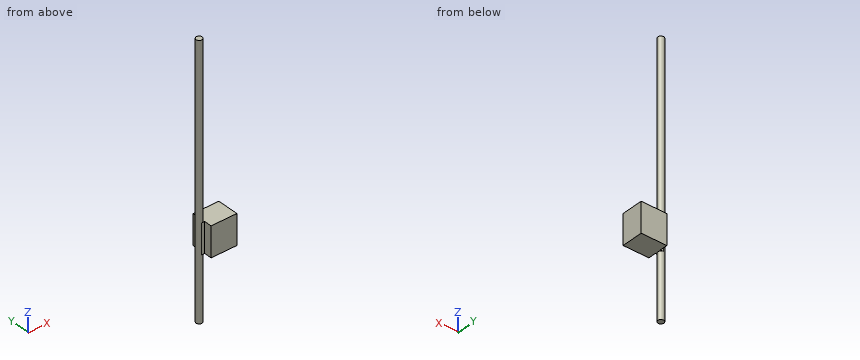
```python
from build123d import *

# Parameters (mm, degrees)
F0_R     = 17.78
F1_DEPTH = 787.4
F2_W     = 152.4
F2_H     = 177.8
F3_DEPTH = 63.5
F5_DEPTH = 177.8


with BuildPart() as f1:
    # F0 (on Top) → F1 (new body, symmetric)
    with BuildSketch(Plane.XY):
        Circle(F0_R)
    extrude(amount=F1_DEPTH, both=True)

    # F2 (on Front) → F3 (join, symmetric)
    with BuildSketch(Plane.XZ):
        with Locations((93.98, -317.5)):
            Rectangle(F2_W, F2_H)
    extrude(amount=F3_DEPTH, both=True)

    # F4 (on face) → F5 (join, through all)
    with BuildSketch(Plane.XY.offset(-228.6)):
        with BuildLine():
            Line((17.78, -17.78), (17.78, 0))
            ThreePointArc((17.78, 0), (12.5723585695, -12.5723585695), (0, -17.78))
            Line((0, -17.78), (17.78, -17.78))
        make_face()
        with BuildLine():
            ThreePointArc((0, 17.78), (12.5723585695, 12.5723585695), (17.78, 0))
            Line((17.78, 0), (17.78, 17.78))
            Line((17.78, 17.78), (0, 17.78))
        make_face()
    extrude(amount=-F5_DEPTH)


solid = f1.part
```
Verification items for the finished model (mm, model axes). Coordinates: 2 decimals unless noted, no trailing zeros. Write each loop counter-clockwise with the first axis right and the second up, starting at its lowest first coordinate (ties: lowest second). Pieces come first, ordered by that corner, then holes. Notation, with made-up numbers: (54, 21) - (107, 21) arc R11 cw to (107, 31) - close; hole circle Ø6 at (70, 45.25). An arc over 180 degrees is marked (long way). One line per question, with ' | ' between items. Start each with the question number.
1. Section check A-A (y = 0). Enter the section's corners in (x, z).
2. Gauge pin test, flat ends, axial feed: P1, Ø5.5, axis at x = 12.5, z = -305.5, coming from the -Y side; P2, Ø8, axis at x = 37, y = -24, coming from the -Z side; P3, Ø1, axis at x = 137, y = 34.5, coming from the +Z side. Record the tip position at first contact, or that the pin passes through.
3. Section check B-B (z = 208). Enter the section's corners in (x, y), plus the area to 3 significant figures.
4. Material ranges on line 1 along Z through (x, y) = (130, 0.5); line 2 along X through (y, z) = (-29.5, -386.5); line 3 along Y through (x, z) = (-3, -126), recorded low to high.
5. Section check C-C (x = 52.5). Enter the section's corners in (y, z), plus the area to 3 significant figures.
Computed values:
1) outline: (-17.78, -787.4) - (17.78, -787.4) - (17.78, -406.4) - (170.18, -406.4) - (170.18, -228.6) - (17.78, -228.6) - (17.78, 787.4) - (-17.78, 787.4) - close
2) P1: y = -17.78 | P2: z = -406.4 | P3: z = -228.6
3) outline: circle Ø35.56 at (0, 0) | area: 993 mm²
4) line 1: -406.4 to -228.6 | line 2: 17.78 to 170.18 | line 3: -17.53 to 17.53
5) outline: (-63.5, -406.4) - (63.5, -406.4) - (63.5, -228.6) - (-63.5, -228.6) - close | area: 22,600 mm²
